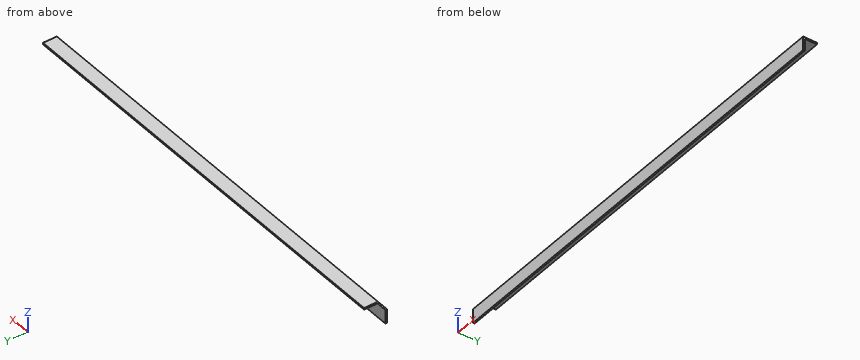
from build123d import *

# Parameters (mm, degrees)
EXTRUDE_1_DEPTH     = 800
SKETCH_2_W          = 22
SKETCH_2_H          = 22
CUT_EXTRUDE_1_DEPTH = 26


with BuildPart() as part:
    # Эскиз1 → Вытянуть-Тонкостенный1 (new body)
    with BuildSketch(Plane(origin=(0, 0, 0), x_dir=(0, 0, -1), z_dir=(1, 0, 0))):
        Polygon((0, 25), (0, 0), (25, 0), (25, 3), (3, 3), (3, 25), align=None)
    extrude(amount=EXTRUDE_1_DEPTH)

    # Эскиз2 → Вырез-Вытянуть1 (cut, through all)
    with BuildSketch(Plane.XY):
        with Locations((11, 14)):
            Rectangle(SKETCH_2_W, SKETCH_2_H)
    extrude(amount=-CUT_EXTRUDE_1_DEPTH, mode=Mode.SUBTRACT)


solid = part.part
Can you work these out from the model? Positions are in its coordinate system, mm. Coordinates: 2 decimals unless noted, no trailing zeros. Order: outer loops, then holes, each group sorted by start corner. A loop starts at its lowest first (then second) coordinate and runs counter-clockwise, first axis right, second up. Notation, with made-up numbers: M 65,-31.5 L 117,-31.5 A30 cw 117,-3.5 Z; hole C -29.75,-8.75 d2. An arc over 180 degrees is marked long. Answer as CSV lines item,"result".
(1) Suppose I cut it at A-A on x = 451.5. Please give me the cut outline in (y, z).
Geometry check:
outline,"M 0,-25 L 3,-25 L 3,-3 L 25,-3 L 25,0 L 0,0 Z"
(2) Suppose I cut it at C-C on y = 7. Please give me the cut outline in (x, z).
Geometry check:
outline,"M 22,-3 L 800,-3 L 800,0 L 22,0 Z"
(3) Please list where these lines run through material, in increasing order: L1, parallel to Z at x = 185.5, y = 22.75; L2, parallel to Y at x = 238.5, z = -8.5; L3, parallel to X at y = 19, z = -0.75.
Geometry check:
L1,"-3 to 0"
L2,"0 to 3"
L3,"22 to 800"
(4) I'm going to push flat-ended pins straight in: pin 1 (2 mm diameter, centred on x = 487.5, y = 6.5, fed in from -Z); pin 2 (1.5 mm diameter, centred on y = 12.5, z = -1, fed in from -X); pin 3 (1 mm diameter, centred on x = 530, z = -4.5, fed in from +Y). Where does each tip first touch, or does it pass through?
Geometry check:
pin 1,"z = -3"
pin 2,"x = 22"
pin 3,"y = 3"
(5) Suppose I cut it at B-B on z = -13. Please give me the cut outline in (x, y).
Geometry check:
outline,"M 0,0 L 800,0 L 800,3 L 0,3 Z"
